Autodesk Fusion 360 part; units mm, degrees
sketch "Sketch1" plane through (0, 0, 0) normal (0, 1, 0) x (1, 0, 0)
  circle A0 centre (-139, -97.5) radius 1.5
  circle A1 centre (139, -97.5) radius 1.5
  circle A2 centre (139, 97.5) radius 1.5
  circle A3 centre (-139, 97.5) radius 1.5
  line L0 (139, -97.5) -> (139, 97.5) construction
  line L1 (139, 97.5) -> (-139, 97.5) construction
  line L2 (-139, 97.5) -> (-139, -97.5) construction
  line L3 (-139, -97.5) -> (139, -97.5) construction
  line L4 (0, -97.5) -> (0, 97.5) construction
  line L5 (139, 0) -> (-139, 0) construction
  circle A4 centre (-139, -97.5) radius 4
  circle A5 centre (-139, 97.5) radius 4
  circle A6 centre (139, 97.5) radius 4
  circle A7 centre (139, -97.5) radius 4
  line L6 (-143, -97.5) -> (-135, -97.5)
  line L7 (-135, -97.5) -> (-135, 97.5)
  line L8 (-135, 97.5) -> (-143, 97.5)
  line L9 (-143, 97.5) -> (-143, -97.5)
  line L10 (143, -97.5) -> (135, -97.5)
  line L11 (135, -97.5) -> (135, 97.5)
  line L12 (135, 97.5) -> (143, 97.5)
  line L13 (143, 97.5) -> (143, -97.5)
  line L14 (-143, -5) -> (143, -5)
  line L15 (143, -5) -> (143, 5)
  line L16 (143, 5) -> (-143, 5)
  line L17 (-143, 5) -> (-143, -5)
  line L18 (-35, -5) -> (-136.2569, -100.4112)
  line L19 (-46.6654, -5) -> (-141.7431, -94.5888)
  line L20 (-136.2569, -100.4112) -> (-141.7431, -94.5888)
  line L21 (35, -5) -> (136.2569, -100.4112)
  line L22 (46.6654, -5) -> (141.7431, -94.5888)
  line L23 (136.2569, -100.4112) -> (141.7431, -94.5888)
  line L24 (-35, 5) -> (-136.2569, 100.4112)
  line L25 (-46.6654, 5) -> (-141.7431, 94.5888)
  line L26 (46.6654, 5) -> (141.7431, 94.5888)
  line L27 (35, 5) -> (136.2569, 100.4112)
  line L28 (136.2569, 100.4112) -> (141.7431, 94.5888)
  line L29 (-136.2569, 100.4112) -> (-141.7431, 94.5888)
  circle A8 centre (-14, 0) radius 1.25
  circle A9 centre (14, 0) radius 1.25
  dimension "d1" = 3
  dimension "d2" = 3
  dimension "d3" = 3
  dimension "d4" = 3
  dimension "d5" = 278
  dimension "d6" = 195
  dimension "d7" = 8
  dimension "d8" = 8
  dimension "d9" = 8
  dimension "d10" = 8
  dimension "d11" = 5
  dimension "d12" = 5
  dimension "d13" = 35
  dimension "d14" = 2.5
  dimension "d15" = 2.5
  dimension "d16" = 14
  dimension "d17" = 14
extrude "Extrude1" add sketch "Sketch1" along normal blind 8.5 contours A0 A4 L6 L20 | A0 A4 L6 L20 | A0 A4 L6 L20 | A0 A4 L6 L20 | A4 L7 L14 L18 L19 | A4 L7 L19 | A4 L7 L9 L14 L19 | L7 L11 L14 L16 | L7 L9 L14 L16 L17 | A7 L11 L14 L21 L22 | A5 L7 L9 L16 L25 | A1 A7 L10 L23 | A1 A7 L10 L23 | A5 L7 L25 | A5 L7 L16 L24 L25 | A3 A5 L8 L29 | A3 A5 L8 L29 | A7 L11 L13 L14 L22 | L11 L13 L14 L15 L16 | A7 L11 L22 | A1 A7 L10 L23 | A1 A7 L10 L23 | A3 A5 L8 L29 | A3 A5 L8 L29 | A6 L11 L13 L16 L26 | A6 L11 L16 L26 L27 | A6 L11 L26 | A2 A6 L12 L28 | A2 A6 L12 L28 | A2 A6 L12 L28 | A2 A6 L12 L28
equation "d2 = d1"
equation "d3 = d2"
equation "d4 = d1"
equation "d8 = d7"
equation "d9 = d7"
equation "d10 = d7"
equation "d12 = d11"
equation "d17 = d16"
Part model, mm, in its own coordinate system. A direction names the side the tool comes from. Round coordinates to 2 decimals unless told otherwise and drop trailing zeros. Loops run counter-clockwise (first coordinate to the right, second up) from the corner with the lowest first, then second, coordinate; pieces in that order, holes last. Notation, with made-up numbers: (22.25, -21) - (73.25, -21) arc R23 cw to (73.25, 17) - close; hole circle Ø11 at (23.25, -32). An arc over 180 degrees is marked (long way). Answer as a JSON object with one key per item and string values.
Item 1: Band-saw the part on C-C on x = -60.5. List the corners of the cut face in (y, z).
Output:
{"outline": "(0, -29.03) - (8.5, -29.03) - (8.5, -18.04) - (0, -18.04) - close; (0, -5) - (8.5, -5) - (8.5, 5) - (0, 5) - close; (0, 18.04) - (8.5, 18.04) - (8.5, 29.03) - (0, 29.03) - close"}
Item 2: Pin check, flat tips, straight feed: pin 1 (3.5 mm diameter, centred on x = 139, z = 97.5, fed in from +Y); pin 2 (2.5 mm diameter, centred on x = 92.5, y = 6, fed in from -Z); pin 3 (2.5 mm diameter, centred on x = 1, y = 4.5, fed in from -Z); pin 4 (3 mm diameter, centred on x = -70.5, y = 4.5, fed in from -Z). Stop position of each tip, or through.
Output:
{"pin 1": "y = 8.5", "pin 2": "z = -60.36", "pin 3": "z = -5", "pin 4": "z = -39.86"}
Item 3: Band-saw the part on D-D on x = 1. List the corners of the cut face in (y, z), plus the area to 3 significant figures.
Output:
{"outline": "(0, -5) - (8.5, -5) - (8.5, 5) - (0, 5) - close", "area": "85.0 mm2"}
Item 4: Band-saw the part on B-B on y = 1.5. State how many separate pieces and enclosed holes the cut face has, plus the area to 3 significant figures.
Output:
{"separate pieces": "1", "enclosed holes": "10", "area": "10,000 mm2"}
Item 5: Wall check: L1, parallel to Z at x = -139, y = 4.25; L2, parallel to X at y = 3.25, z = 0; L3, parallel to Z at x = 14, y = 1.5. Give the ranges that are in metal, low to high.
Output:
{"L1": "-101.5 to -99, -96 to 96, 99 to 101.5", "L2": "-143 to -15.25, -12.75 to 12.75, 15.25 to 143", "L3": "-5 to -1.25, 1.25 to 5"}
Item 6: Pull direction Z, two halves, no side cores. Call faces 1 (the face through (-90.21, 4.19, -46.03)), 2 (the face through (84.92, 4.19, 52.04)), 3 (the face through (-143, 4, -1)), 4 (the face through (90, 4, 5)): pulls with the +Z half, pulls with the -Z half, needs draft (parallel to the pull), parting line crosses it, or undercut.
Output:
{"face 1": "undercut", "face 2": "pulls with the +Z half", "face 3": "needs draft", "face 4": "undercut"}
Item 7: Band-saw the part on A-A on z = -84. List the corners of the cut face in (x, y).
Output:
{"outline": "(-143, 0) - (-135, 0) - (-135, 8.5) - (-143, 8.5) - close; (-130.51, 0) - (-118.84, 0) - (-118.84, 8.5) - (-130.51, 8.5) - close; (118.84, 0) - (130.51, 0) - (130.51, 8.5) - (118.84, 8.5) - close; (135, 0) - (143, 0) - (143, 8.5) - (135, 8.5) - close"}
Item 8: Tool access for faces 5 (the face through (0, 4, -5)), 6 (the face through (-84.92, 4.19, 52.04)), 7 (the face through (10, 8.5, 0)), 8 (the face through (-91, 4, 5)): list every direction of +Z, -Z, +X, -X, +Y, -Y with a clear straight run to the whole face (end or side of a thin tool).
Output:
{"face 5": "-Z, +Y, -Y", "face 6": "+Z, +Y, -Y", "face 7": "+Z, -Z, +X, -X, +Y", "face 8": "+Y, -Y"}
